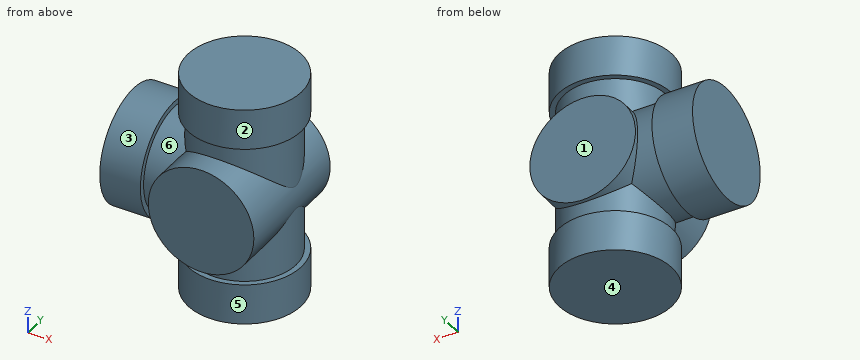
from build123d import *

# Parameters (mm, degrees)
SKETCH002_R  = 19.5
PAD_DEPTH    = 20.33
PAD001_DEPTH = 27


with BuildPart() as part:
    # Sketch → Revolution (revolve)
    with BuildSketch(Plane.XZ):
        Polygon((0, -41), (21, -41), (21, -26), (19, -26), (19, 26), (21, 26), (21, 41), (0, 41), align=None)
    revolve(axis=Axis((0, 0, 0), (0, 0, 1)))

    # Sketch001 → Revolution001 (revolve)
    with BuildSketch(Plane.XZ):
        Polygon((0, 0), (0, -19), (-26, -19), (-26, -21), (-41, -21), (-41, 0), align=None)
    revolve(axis=Axis((0, 0, 0), (1, 0, 0)))

    # Sketch002 → Pad (new body)
    with BuildSketch(Plane.XZ):
        Circle(SKETCH002_R)
    extrude(amount=-PAD_DEPTH)

    # Sketch002 → Pad001 (join)
    with BuildSketch(Plane.XZ):
        Circle(SKETCH002_R)
    extrude(amount=PAD001_DEPTH)


solid = part.part
Geometry check sheet. Reference: the model listing, model coordinates, mm. Face numbers are marked on the shaded views. A direction names the side the tool comes from. Give positions to 0.01 mm unless a question says otherwise; leave off trailing zeros. Order: outer loops, then holes, each group sorted by start corner. A loop starts at its lowest first (then second) coordinate and runs counter-clockwise, first axis right, second up. Notation, with made-up numbers: M 38,-31.75 L 86,-31.75 A22 ccw 86,-4.75 Z; hole C 16,72.5 d9. An arc over 180 degrees is marked long. Use a Markdown table: item, result.
Item 1: Depth check by flat-ended pin: P1, Ø1.5, axis at y = -18.5, z = 18, coming from the +X side; P2, Ø5, axis at x = 14.5, z = 19, coming from the -Y side; P3, Ø1, axis at y = 16, z = 14, coming from the -X side; P4, Ø1.5, axis at x = 12.5, y = -20.5, coming from the -Z side. Enter the tip coordinate at first touch or a pass-through.
Answers follow:
| item | result |
|---|---|
| P1 | stops at x = 9.09 |
| P2 | stops at y = -14.73 |
| P3 | stops at x = -41 |
| P4 | stops at z = -15.56 |
Item 2: Section check B-B (y = 0). Record the cut outline in (x, z).
Answers follow:
| item | result |
|---|---|
| outline | M -41,-21 L -26,-21 L -26,-19 L -19,-19 L -19,-26 L -21,-26 L -21,-41 L 21,-41 L 21,-26 L 19,-26 L 19,-4.39 A19.5 ccw 19,4.39 L 19,26 L 21,26 L 21,41 L -21,41 L -21,26 L -19,26 L -19,19 L -26,19 L -26,21 L -41,21 Z |
Item 3: Tool access check on the marked faces 1, 2 and 3. Record the directions out of +Z, -Z, +X, -X, +Y, -Y that give a thin tool (end or side, any length) a straight path to the whole face; none if there is none.
Answers follow:
| item | result |
|---|---|
| face 1 | +X, +Y |
| face 2 | +Z |
| face 3 | -X |
Item 4: Draft check along Z on the marked faces 4, 5 and 6. Enter one of: +Z half, -Z half, draft (parallel to the pull), parting line (faces both ways), or undercut.
Answers follow:
| item | result |
|---|---|
| face 4 | -Z half |
| face 5 | draft |
| face 6 | undercut |
Item 5: Section check A-A (x = 0). Record the cut outline in (y, z), and give its area (3 significant figures).
Answers follow:
| item | result |
|---|---|
| outline | M -27,-19.5 L -19,-19.5 L -19,-26 L -21,-26 L -21,-41 L 21,-41 L 21,-26 L 19,-26 L 19,-19.5 L 20.33,-19.5 L 20.33,19.5 L 19,19.5 L 19,26 L 21,26 L 21,41 L -21,41 L -21,26 L -19,26 L -19,19.5 L -27,19.5 Z |
| area | 3,600 mm2 |
Item 6: Material ranges on line 1 along Z through (x, y) = (16, 11.5); line 2 along Y through (x, z) = (-14, -13.5); line 3 along Z through (x, y) = (15, 13.5), recorded low to high.
Answers follow:
| item | result |
|---|---|
| line 1 | z = -41 to -26, -11.15 to 11.15, 26 to 41 |
| line 2 | y = -27 to 20.33 |
| line 3 | z = -41 to -26, -12.46 to 12.46, 26 to 41 |
Item 7: Section check D-D (y = 8). Record the cut outline in (x, z).
Answers follow:
| item | result |
|---|---|
| outline | M -41,-19.42 L -26,-19.42 L -26,-17.23 L -17.23,-17.23 L -17.23,-26 L -19.42,-26 L -19.42,-41 L 19.42,-41 L 19.42,-26 L 17.23,-26 L 17.23,-9.12 A19.5 ccw 17.23,9.12 L 17.23,26 L 19.42,26 L 19.42,41 L -19.42,41 L -19.42,26 L -17.23,26 L -17.23,17.23 L -26,17.23 L -26,19.42 L -41,19.42 Z |
Item 8: Section check C-C (z = 0). Record the cut outline in (x, y).
Answers follow:
| item | result |
|---|---|
| outline | M -41,-21 L -26,-21 L -26,-19 L -19.5,-19 L -19.5,-27 L 19.5,-27 L 19.5,20.33 L -19.5,20.33 L -19.5,19 L -26,19 L -26,21 L -41,21 Z |
